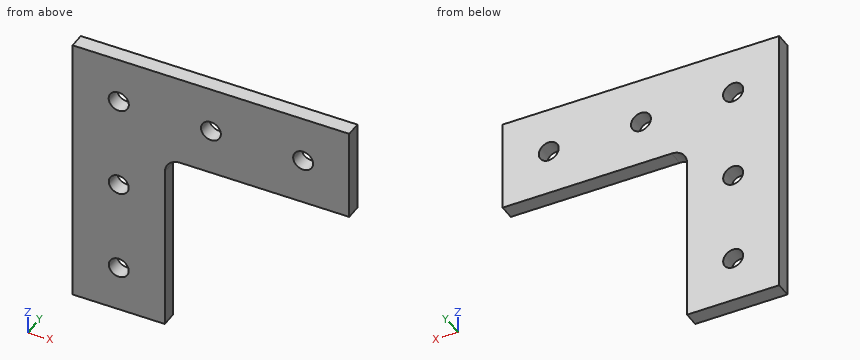
```python
from build123d import *

# Parameters (mm, degrees)
SKETCH1_R           = 4.1656
SKETCH1_R_2         = 4.1148
BOSS_EXTRUDE1_DEPTH = 6.35


with BuildPart() as part:
    # Sketch1 → Boss-Extrude1 (new body)
    with BuildSketch(Plane(origin=(0, 0, 0), x_dir=(1, 0, 0), z_dir=(0, 1, 0))):
        with BuildLine():
            Line((-94.42173913, 44.607763975), (-94.42173913, -69.692236025))
            Line((-94.42173913, -69.692236025), (19.87826087, -69.692236025))
            Line((19.87826087, -69.692236025), (19.87826087, -31.592236025))
            Line((19.87826087, -31.592236025), (-49.97173913, -31.592236025))
            ThreePointArc((-49.97173913, -31.592236025), (-54.461867191, -29.732364085), (-56.32173913, -25.242236025))
            Line((-56.32173913, -25.242236025), (-56.32173913, 44.607763975))
            Line((-56.32173913, 44.607763975), (-94.42173913, 44.607763975))
        make_face()
        with Locations(Location((-75.37173913, -50.642236025, 0), (0, 0, 270))):
            Circle(SKETCH1_R, mode=Mode.SUBTRACT)
        with Locations(Location((0.82826087, -50.642236025, 0), (0, 0, 270))):
            Circle(SKETCH1_R_2, mode=Mode.SUBTRACT)
        with Locations(Location((-37.27173913, -50.642236025, 0), (0, 0, 270))):
            Circle(SKETCH1_R_2, mode=Mode.SUBTRACT)
        with Locations(Location((-75.37173913, 25.557763975, 0), (0, 0, 270))):
            Circle(SKETCH1_R_2, mode=Mode.SUBTRACT)
        with Locations(Location((-75.37173913, -12.542236025, 0), (0, 0, 270))):
            Circle(SKETCH1_R_2, mode=Mode.SUBTRACT)
    extrude(amount=BOSS_EXTRUDE1_DEPTH)


solid = part.part
```
The listing builds one solid part. Answer for the finished solid, in the listing's coordinates (mm). Coordinates: 2 decimals unless noted, no trailing zeros. Write each loop counter-clockwise with the first axis right and the second up, starting at its lowest first coordinate (ties: lowest second). Pieces come first, ordered by that corner, then holes. Notation, with made-up numbers: (16.25, 71.25) - (63.25, 71.25) arc R23 ccw to (63.25, 82.25) - close; hole circle Ø6 at (-30.5, 9). An arc over 180 degrees is marked (long way). Return JSON: item names as keys, results as strings. Group by question number.
1. A cutting plane is placed at C-C, the plane x = -17. Determine the outline of the cut face in (y, z), plus the area to 3 significant figures.
2. Straight lines are drawn through the part: L1, parallel to Z at x = -75, y = 6; L2, parallel to X at y = 1.75, z = 49; L3, parallel to Z at x = -26.5, y = 4.75. For each, find the intervals that lie inside material, in ascending order.
3. A cutting plane is placed at A-A, the plane y = 1.75. Determine the outline of the cut face in (x, z).
4. Given pin 1 (5 mm diameter, centred on x = -75.37, z = -25.56, fed in from -Y); pin 2 (9.5 mm diameter, centred on x = 0.83, z = 50.64, fed in from -Y); pin 3 (3 mm diameter, centred on y = 2.5, z = -1, fed in from +X), each flat-ended and moving along its own axis, determine where each tip first touches the part or whether it passes through.
5. A cutting plane is placed at B-B, the plane z = -37. Determine the outline of the cut face in (x, y), plus the area to 3 significant figures.
Ans:
{
 "1": {"outline": "(0, 31.59) - (6.35, 31.59) - (6.35, 69.69) - (0, 69.69) - close", "area": "242 mm²"},
 "2": {"L1": "-44.61 to -29.66, -21.46 to 8.44, 16.64 to 46.49, 54.79 to 69.69", "L2": "-94.42 to -79.2, -71.54 to -41.04, -33.5 to -2.94, 4.6 to 19.88", "L3": "31.59 to 69.69"},
 "3": {"outline": "(-94.42, -44.61) - (-56.32, -44.61) - (-56.32, 25.24) arc R6.35 cw to (-49.97, 31.59) - (19.88, 31.59) - (19.88, 69.69) - (-94.42, 69.69) - close; hole circle Ø8.33 at (-75.37, 50.64); hole circle Ø8.23 at (-75.37, -25.56); hole circle Ø8.23 at (-75.37, 12.54); hole circle Ø8.23 at (-37.27, 50.64); hole circle Ø8.23 at (0.83, 50.64)"},
 "4": {"pin 1": "through", "pin 2": "y = 0", "pin 3": "x = -56.32"},
 "5": {"outline": "(-94.42, 0) - (-56.32, 0) - (-56.32, 6.35) - (-94.42, 6.35) - close", "area": "242 mm²"}
}
